Part model, mm, in its own coordinate system. A direction names the side the tool comes from. Give positions to 0.01 mm unless a question says otherwise; leave off trailing zeros. Write each loop counter-clockwise with the first axis right and the second up, starting at its lowest first coordinate (ties: lowest second). Pieces come first, ordered by that corner, then holes. Notation, with made-up numbers: M 71,-27.5 L 108,-27.5 A27 cw 108,7.5 Z; hole C -33,-19.5 d6. An arc over 180 degrees is marked long. Answer as CSV lines item,"result". Start each with the question number.
Item 1: 3-axis set-ups, long thin cutter, end or side, ignore diameter. For faces 5 (the flat face through (25.4, 13, 31)), 6 (the flat face through (-0.6, 65.8, 37.28)), 7 (the cylindrical face through (11.5, 30.1, 35)), 8 (the cylindrical face through (10.018, 4.184, 45.53)): which of +Z, -Z, +X, -X, +Y, -Y reach the whole face in a straight line?
Item 2: Band-saw the part on B-B, the plane y = 45.5. List the corners of the cut face in (x, z).
Item 3: Wall check: L1, parallel to Y at x = 12.7, z = 17; L2, parallel to Y at x = 12, z = 59 (3 decimals). Give the ranges that are in metal, low to high. Write a range as from..to.
Item 4: Two-plate mould, pull along Y, no slides. Class faces 1 (the cylindrical face through (12.86, 0.48, 63.05)), 2 (the cylindrical face through (11.047, 47.447, 31.858)), 3 (the flat face through (25.56, 65.8, 36.52)), 4 (the cylindrical face through (24.92, 24.95, 32.17)): +Y half, -Y half, draft (parallel to the pull), parting line (faces both ways), or undercut.
Item 5: Band-saw the part on A-A, the plane z = 8. List the corners of the cut face in (x, y) (1 decimal), then the cut area to 3 significant figures.
Item 6: Pin check, flat tips, straight feed: pin 1 (8 mm diameter, centred on y = 26, z = 51.5, fed in from +X); pin 2 (11 mm diameter, centred on y = 11, z = 23, fed in from -X); pin 3 (5.5 mm diameter, centred on x = 9, y = 11, fed in from +Z). Stop position of each tip, or through.
from build123d import *

# Parameters (mm, degrees)
SKETCH1_W           = 25.4
SKETCH1_H           = 25.4
BOSS_EXTRUDE1_DEPTH = 63.5
SKETCH4_R           = 9.525
BOSS_EXTRUDE2_DEPTH = 9.525
SKETCH5_R           = 12.7
BOSS_EXTRUDE3_DEPTH = 25.4
BOSS_EXTRUDE4_DEPTH = 12.7
FILLET1_R           = 1.5875


with BuildPart() as part:
    # Sketch1 → Boss-Extrude1 (new body)
    with BuildSketch(Plane.XY):
        with Locations((12.7, 12.7)):
            Rectangle(SKETCH1_W, SKETCH1_H)
    extrude(amount=BOSS_EXTRUDE1_DEPTH)

    # Sketch2 → 1/2 NPT Tapped Hole1 (revolve, cut)
    with BuildSketch(Plane(origin=(12.7, 12.7, 63.5), x_dir=(0, -1, 0), z_dir=(1, 0, 0))):
        Polygon((0, 0), (0, 27.970543693), (8.9281, 22.606), (8.9281, 13.462), (9.479726792, 13.462), (9.8827971, 0), align=None)
    revolve(axis=Axis((12.7, 12.7, 69.85), (0, 0, -1)), mode=Mode.SUBTRACT)

    # Sketch4 → Boss-Extrude2 (add)
    with BuildSketch(Plane(origin=(0, 25.4, 0), x_dir=(1, 0, 0), z_dir=(0, 1, 0))):
        with Locations((12.7, -44.45)):
            Circle(SKETCH4_R)
    extrude(amount=BOSS_EXTRUDE2_DEPTH)

    # Sketch5 → Boss-Extrude3 (add)
    with BuildSketch(Plane(origin=(0, 34.925, 0), x_dir=(1, 0, 0), z_dir=(0, 1, 0))):
        with Locations((12.7, -44.45)):
            Circle(SKETCH5_R)
    extrude(amount=BOSS_EXTRUDE3_DEPTH)

    # Sketch6 → Boss-Extrude4 (add)
    with BuildSketch(Plane(origin=(0, 60.325, 0), x_dir=(1, 0, 0), z_dir=(0, 1, 0))):
        Polygon((3.422327472, -29.674263649), (-4.734999304, -45.096831921), (4.542673224, -59.872568273), (21.977672528, -59.225736351), (30.134999304, -43.803168079), (20.857326776, -29.027431727), align=None)
    extrude(amount=BOSS_EXTRUDE4_DEPTH)

    # Sketch7 → 1/2 NPT Tapped Hole2 (revolve, cut)
    with BuildSketch(Plane(origin=(12.7, 12.7, 0), x_dir=(0, 1, 0), z_dir=(1, 0, 0))):
        Polygon((0, 0), (0, 27.970543693), (8.9281, 22.606), (8.9281, 13.462), (9.479726792, 13.462), (9.8827971, 0), align=None)
    revolve(axis=Axis((12.7, 12.7, -6.35), (0, 0, 1)), mode=Mode.SUBTRACT)

    # Fillet1
    fillet1_edges = [part.edges().sort_by_distance(p)[0] for p in [
        (25.4, 12.7, 63.5),
        (12.7, 25.4, 63.5),
        (12.139827124, 73.025, 29.350847688),
        (-0.656335916, 73.025, 37.385547785),
        (-0.09616304, 73.025, 52.484700097),
        (13.260172876, 73.025, 59.549152312),
        (26.056335916, 73.025, 51.514452215),
        (25.49616304, 73.025, 36.415299903),
        (0, 12.7, 63.5),
        (12.7, 25.4, 0),
        (25.4, 12.7, 0),
        (12.7, 0, 0),
        (0, 12.7, 0),
        (12.7, 0, 63.5),
        (0, 25.4, 31.75),
        (25.4, 25.4, 31.75),
        (25.4, 0, 31.75),
        (0, 0, 31.75),
    ]]
    fillet(fillet1_edges, radius=FILLET1_R)


solid = part.part
Output:
1,face 5,"+Z, -Z, +X, -Y"
1,face 6,"-Z, -X, +Y"
1,face 7,"none"
1,face 8,"+Z"
2,outline,"C 12.7,44.45 d25.4"
3,L1,"0..3.77, 21.63..25.4"
3,L2,"0..2.977, 22.423..25.4, 60.325..72.677"
4,face 1,"-Y half"
4,face 2,"undercut"
4,face 3,"draft"
4,face 4,"undercut"
5,outline,"M 0,1.6 A1.6 ccw 1.6,0 L 23.8,0 A1.6 ccw 25.4,1.6 L 25.4,23.8 A1.6 ccw 23.8,25.4 L 1.6,25.4 A1.6 ccw 0,23.8 Z; hole C 12.7,12.7 d19.3"
5,area,"351 mm²"
6,pin 1,"x = 25.4"
6,pin 2,"x = 0"
6,pin 3,"z = 39.63"
